from build123d import *

# Parameters (mm, degrees)
SKETCH1_R               = 2.15
BOSS_EXTRUDE1_DEPTH     = 31
CUT_EXTRUDE1_REACH      = 45.327
SKETCH2_W               = 57
SKETCH2_H               = 12
SKETCH7_R               = 1.4
CUT_EXTRUDE2_DEPTH      = 9
CUT_EXTRUDE3_DEPTH      = 68.771693944
FILLET1_R               = 2
CUT_EXTRUDE4_DEPTH      = 39.007433483
CUT_EXTRUDE4_DEPTH_BACK = 39.007433483
SKETCH9_W               = 62
SKETCH9_H               = 45.1
SKETCH9_W_2             = 61
SKETCH9_H_2             = 43.1


with BuildPart() as part:
    # Sketch1 → Boss-Extrude1 (new, symmetric)
    with BuildSketch(Plane(origin=(0, 0, 0), x_dir=(0, 0, -1), z_dir=(1, 0, 0))):
        with BuildLine():
            Line((-4.25, 0), (-4.25, -4))
            ThreePointArc((-4.25, -4), (-4.105356672, -4.642657212), (-3.699322277, -5.161372987))
            Line((-3.699322277, -5.161372987), (-2.000677723, -6.549868444))
            ThreePointArc((-2.000677723, -6.549868444), (-1.594643328, -7.068584218), (-1.45, -7.71124143))
            Line((-1.45, -7.71124143), (-1.45, -21))
            Line((-1.45, -21), (17.55, -21))
            Line((17.55, -21), (8.093870957, -13.612062296))
            Line((8.093870957, -13.612062296), (4.101919606, 1.112095114))
            ThreePointArc((4.101919606, 1.112095114), (-0.560955289, 4.212817248), (-4.25, 0))
        make_face()
        Circle(SKETCH1_R, mode=Mode.SUBTRACT)
    extrude(amount=BOSS_EXTRUDE1_DEPTH, both=True)

    # Cut-Extrude1: up to this plane
    cut_extrude1_end = Plane(origin=(31, -13.612062296, -8.093870957), z_dir=(0, -0.26166943856052705, 0.9651575544559649))
    # Sketch2 → Cut-Extrude1 (cut, up to the surface)
    with BuildSketch(Plane.XY.offset(4.25), mode=Mode.PRIVATE) as cut_extrude1_sk1:
        with Locations((0, -1.75)):
            Rectangle(SKETCH2_W, SKETCH2_H)
    cut_extrude1_tool1 = split(extrude(cut_extrude1_sk1.sketch, amount=-CUT_EXTRUDE1_REACH, mode=Mode.PRIVATE), bisect_by=cut_extrude1_end, keep=Keep.BOTH, mode=Mode.PRIVATE)
    add(cut_extrude1_tool1.solids().sort_by_distance((0, -1.75, 4.25))[0], mode=Mode.SUBTRACT)

    # Sketch7 → Cut-Extrude2 (cut)
    with BuildSketch(Plane.XY.offset(4.25)):
        with Locations((-12.9, -14.375)):
            Circle(SKETCH7_R)
        with Locations(Location((12.9, -14.375, 0), (0, 0, 90))):
            Circle(SKETCH7_R)
    extrude(amount=-CUT_EXTRUDE2_DEPTH, mode=Mode.SUBTRACT)

    # Sketch8 → Cut-Extrude3 (cut, through all)
    with BuildSketch(Plane(origin=(31, 0, 0), x_dir=(0, 0, -1), z_dir=(1, 0, 0))):
        with BuildLine():
            Line((-1.45, -7.71124143), (6.504573393, -7.75))
            Line((6.504573393, -7.75), (4.101919606, 1.112095114))
            ThreePointArc((4.101919606, 1.112095114), (-0.560955289, 4.212817248), (-4.25, 0))
            Line((-4.25, 0), (-4.25, -4))
            ThreePointArc((-4.25, -4), (-4.105356672, -4.642657212), (-3.699322277, -5.161372987))
            Line((-3.699322277, -5.161372987), (-2.000677723, -6.549868444))
            ThreePointArc((-2.000677723, -6.549868444), (-1.594643328, -7.068584218), (-1.45, -7.71124143))
        make_face()
    extrude(amount=-CUT_EXTRUDE3_DEPTH, mode=Mode.SUBTRACT)

    # Fillet1
    fillet1_edges = [part.edges().sort_by_distance(p)[0] for p in [
        (31, -14.355620715, 1.45),
        (-31, -14.355620715, 1.45),
    ]]
    fillet(fillet1_edges, radius=FILLET1_R)

    # Sketch9 → Cut-Extrude4 (cut, two sides: drawn at the far end of the back side and taken through both)
    with BuildSketch(Plane(origin=(0, -7.75, 0), x_dir=(1, 0, 0), z_dir=(0, 1, 0)).offset(-CUT_EXTRUDE4_DEPTH_BACK)):
        Rectangle(SKETCH9_W, SKETCH9_H)
        Rectangle(SKETCH9_W_2, SKETCH9_H_2, mode=Mode.SUBTRACT)
    extrude(amount=CUT_EXTRUDE4_DEPTH + CUT_EXTRUDE4_DEPTH_BACK, mode=Mode.SUBTRACT)


solid = part.part
Part model, mm, in its own coordinate system. A direction names the side the tool comes from. Give positions to 0.01 mm unless a question says otherwise; leave off trailing zeros. Loops run counter-clockwise (first coordinate to the right, second up) from the corner with the lowest first, then second, coordinate; pieces in that order, holes last.
(1) Band-saw the part on D-D (x = -23). Write the cut outline in (y, z), and give its area (3 significant figures).
Return value:
outline: (-21, -17.55) - (-13.61, -8.09) - (-7.75, -6.5) - (-7.75, 1.45) - (-21, 1.45) - close
area: 157 mm2
(2) Pull direction X, two halves, no side cores. Call faces 3 (the cylindrical face through (29.81, -14.45, 1.28)), 4 (the cylindrical face through (-12.147, -13.195, -1.607)), 5 (the cylindrical face through (-29.81, -14.45, 1.28)): pulls with the +X half, pulls with the -X half, needs draft (parallel to the pull), parting line crosses it, or undercut.
Return value:
face 3: pulls with the +X half
face 4: undercut
face 5: pulls with the -X half
(3) Drill centre lines: line 1 along Y through (x, z) = (-12.9, 0.25) (3 decimals); line 2 along X through (y, z) = (-15.5, -2.25); line 3 along Y through (x, z) = (-11, 0.5). Where is each one in solid material? Low to high.
Return value:
line 1: y = -21 to -15.775, -12.975 to -7.75
line 2: x = -30.5 to -13.73, -12.07 to 12.07, 13.73 to 30.5
line 3: y = -21 to -7.75
(4) Band-saw the part on A-A (z = -2). Write the cut outline in (x, y) (3 decimals), and give its area (3 significant figures).
Return value:
outline: (-30.5, -21) - (30.5, -21) - (30.5, -7.728) - (28.5, -7.728) - (28.5, -7.75) - (-28.5, -7.75) - (-28.5, -7.728) - (-30.5, -7.728) - close; hole circle Ø2.8 at (-12.9, -14.375); hole circle Ø2.8 at (12.9, -14.375)
area: 796 mm2
(5) Band-saw the part on B-B (x = 12.9). Write the cut outline in (y, z) (3 decimals), and give its area (3 significant figures).
Return value:
outline: (-21, -17.55) - (-13.612, -8.094) - (-7.75, -6.505) - (-7.75, 1.45) - (-12.975, 1.45) - (-12.975, -4.75) - (-15.775, -4.75) - (-15.775, 1.45) - (-21, 1.45) - close
area: 139 mm2
(6) 3-axis set-ups, long thin cutter, end or side, ignore diameter. For faces 1 (the flat face through (-13, -14, -4.75)), 2 (the flat face through (30.5, -16, -6)): which of +Z, -Z, +X, -X, +Y, -Y reach the whole face in a straight line?
Return value:
face 1: +Z
face 2: +Z, -Z, +X, +Y, -Y
(7) Band-saw the part on C-C (y = -16.75). Write the cut outline in (x, z).
Return value:
outline: (-30.5, -12.11) - (30.5, -12.11) - (30.5, 0.77) arc R2 ccw to (29, 1.45) - (-29, 1.45) arc R2 ccw to (-30.5, 0.77) - close
(8) Pin check, flat tips, straight feed: pin 1 (3 mm diameter, centred on x = -23.5, z = -6, fed in from +Y); pin 2 (1.7 mm diameter, centred on x = -12.9, y = -14.375, fed in from +Z). Stop position of each tip, or through.
Return value:
pin 1: stops at y = -7.75
pin 2: stops at z = -4.75
